Model file for the job. Use its own axes, mm. Coordinates: 2 decimals unless noted, no trailing zeros. Write each loop counter-clockwise with the first axis right and the second up, starting at its lowest first coordinate (ties: lowest second). Pieces come first, ordered by that corner, then holes. Notation, with made-up numbers: M 62,-32.75 L 119,-32.75 A12 cw 119,-22.75 Z; hole C -34,-35.5 d7. An arc over 180 degrees is marked long. Put each result on its own line as item: value. Start each with the question number.
Q1. Cut at D-D (x = -5.5). Write the cut outline in (y, z), then the cut area to 3 significant figures.
Q2. Pull direction Y, two halves, no side cores. Call faces 1 (the flat face through (-2, 3, 7)), 2 (the cylindrical face through (-4.85, 16.76, 11.92)), 3 (the flat face through (-22.9, 22.9, 7.4)): pulls with the +Y half, pulls with the -Y half, needs draft (parallel to the pull), parting line crosses it, or undercut.
Q3. Cut at B-B (z = 3). Write the cut outline in (x, y).
Q4. Cut at A-A (y = 12.7). Write the cut outline in (x, z), then the cut area to 3 significant figures.
Q5. Drill centre lines: line 1 along Y through (x, z) = (-12.7, 13); line 2 along Z through (x, y) = (-19, 12.7); line 3 along Z through (x, y) = (-1.5, 8.5). Where is each one in solid material? Low to high.
Q6. Drop a flat-ended pin along its axis: pin 1 (1 mm diameter, centred on y = 21, z = 6, fed in from -X). Give the stop position or say it passes through.
Q7. Cut at C-C (x = -18.25). Write the cut outline in (y, z).
```python
from build123d import *

# Parameters (mm, degrees)
SKETCH1_W           = 25.4
SKETCH1_H           = 25.4
BOSS_EXTRUDE1_DEPTH = 15
CHAMFER1_SIZE       = 5
SKETCH2_R           = 6
CUT_EXTRUDE1_DEPTH  = 39.927111375
SKETCH3_R           = 6
CUT_EXTRUDE2_DEPTH  = 39.927111375


with BuildPart() as part:
    # Sketch1 → Boss-Extrude1 (new body)
    with BuildSketch(Plane.XY):
        with Locations((-12.7, 12.7)):
            Rectangle(SKETCH1_W, SKETCH1_H)
    extrude(amount=BOSS_EXTRUDE1_DEPTH)

    # Chamfer1
    chamfer1_edges = [part.edges().sort_by_distance(p)[0] for p in [
        (0, 25.4, 7.5),
        (0, 0, 7.5),
        (-25.4, 0, 7.5),
        (-25.4, 25.4, 7.5),
    ]]
    chamfer(chamfer1_edges, length=CHAMFER1_SIZE)

    # Sketch2 → Cut-Extrude1 (cut, through all)
    with BuildSketch(Plane.XY.offset(15)):
        with Locations((-12.7, 12.7)):
            Circle(SKETCH2_R)
    extrude(amount=-CUT_EXTRUDE1_DEPTH, mode=Mode.SUBTRACT)

    # Sketch3 → Cut-Extrude2 (cut, through all)
    with BuildSketch(Plane(origin=(0, 0, 0), x_dir=(0, 0, -1), z_dir=(1, 0, 0))):
        with Locations((-7.5, 12.7)):
            Circle(SKETCH3_R)
    extrude(amount=-CUT_EXTRUDE2_DEPTH, mode=Mode.SUBTRACT)


solid = part.part
```
Computed values:
1. outline: M 0,0 L 25.4,0 L 25.4,15 L 0,15 Z; hole C 12.7,7.5 d12
1. area: 268 mm2
2. face 1: pulls with the -Y half
2. face 2: undercut
2. face 3: pulls with the +Y half
3. outline: M -25.4,5 L -20.4,0 L -5,0 L 0,5 L 0,8.73 L -8.2,8.73 A6 cw -17.2,8.73 L -25.4,8.73 Z; M -25.4,16.67 L -17.2,16.67 A6 cw -8.2,16.67 L 0,16.67 L 0,20.4 L -5,25.4 L -20.4,25.4 L -25.4,20.4 Z
4. outline: M -25.4,0 L -18.7,0 L -18.7,1.5 L -25.4,1.5 Z; M -25.4,13.5 L -18.7,13.5 L -18.7,15 L -25.4,15 Z; M -6.7,0 L 0,0 L 0,1.5 L -6.7,1.5 Z; M -6.7,13.5 L 0,13.5 L 0,15 L -6.7,15 Z
4. area: 40.2 mm2
5. line 1: 0 to 6.7, 18.7 to 25.4
5. line 2: 0 to 1.5, 13.5 to 15
5. line 3: 0 to 3.22, 11.78 to 15
6. pin 1: x = -25.3
7. outline: M 0,0 L 10.42,0 L 10.42,1.95 A6 cw 10.42,13.05 L 10.42,15 L 0,15 Z; M 14.98,0 L 25.4,0 L 25.4,15 L 14.98,15 L 14.98,13.05 A6 cw 14.98,1.95 Z
